Check sheet for the drawn part. Datum: minimum x, y, z corner. Units: mm. Coordinates: 2 decimals unless noted, no trailing zeros. Loops run counter-clockwise (first coordinate to the right, second up) from the corner with the lowest first, then second, coordinate; pieces in that order, holes last. Notation, with made-up numbers: (36, 1) - (55, 1) arc R19 cw to (55, 7) - close; hole circle Ø6 at (19.5, 65). An arc over 180 degrees is marked (long way). Answer as a JSON object with one key per item and string values. Group by question number.
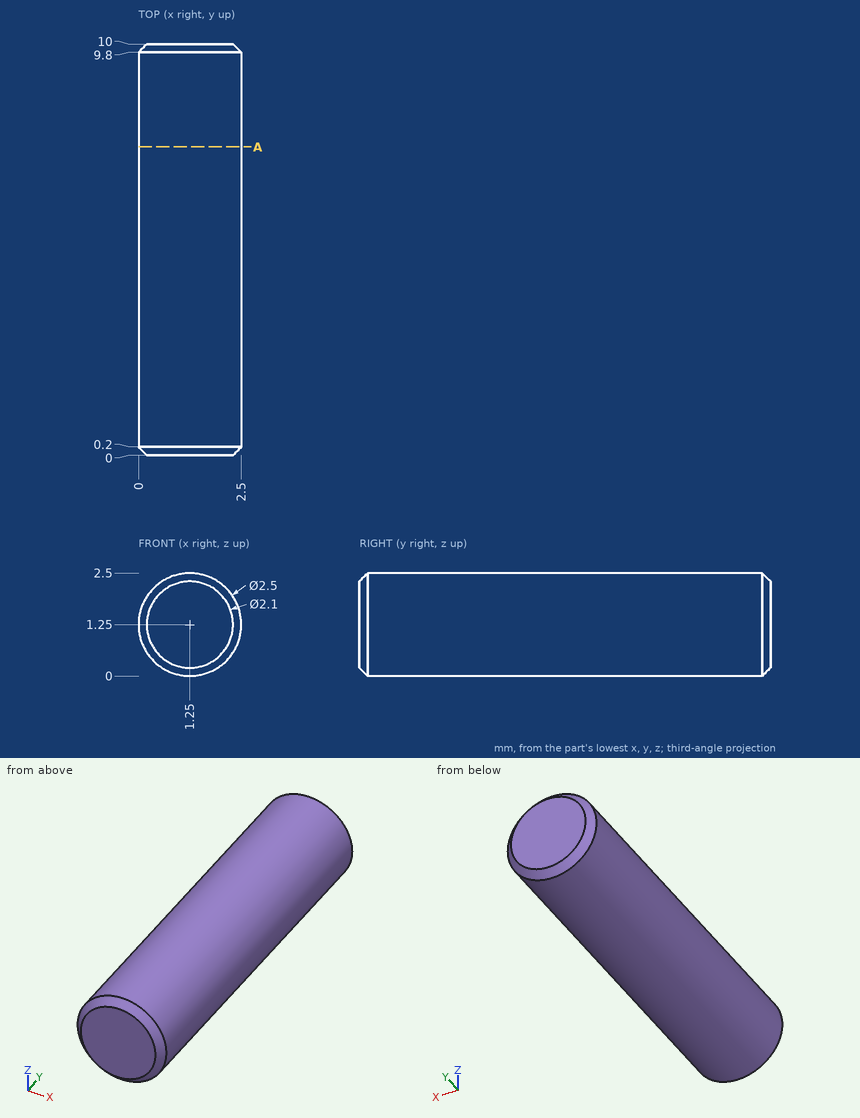
1. Sectioned sample at A-A on y = 7.5. Record the cut outline in (x, z).
2. Material ranges on line 1 (X direction, y = 2.75, z = 1.9); line 2 (X direction, y = 9.5, z = 0.15), recorded low to high.
3. Gauge pin test, flat end, axial feed: pin 1 (1.5 mm diameter, centred on y = 2.5, z = 0.5, fed in from +X). Record the tip position at first contact, or that the pin passes through.
Answers follow:
{
 "1": {"outline": "circle Ø2.5 at (1.25, 1.25)"},
 "2": {"line 1": "x = 0.18 to 2.32", "line 2": "x = 0.66 to 1.84"},
 "3": {"pin 1": "stops at x = 2.5"}
}
